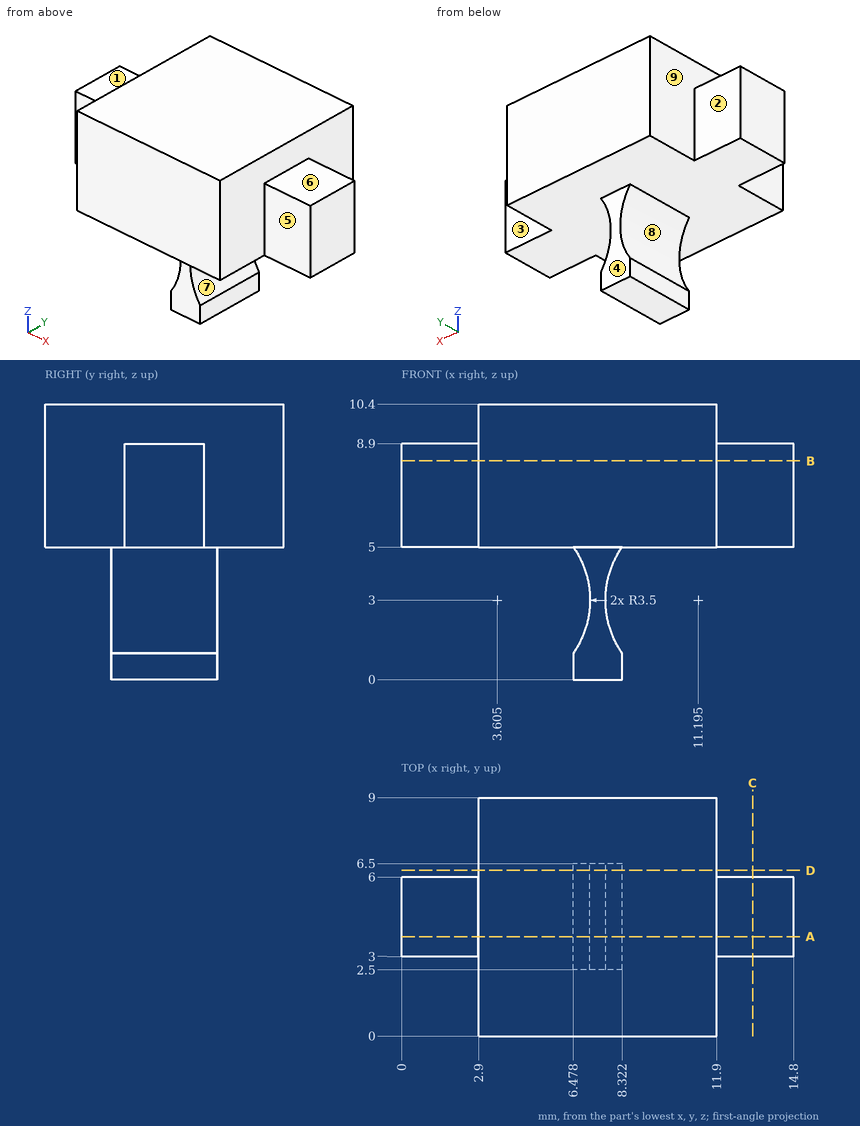
Geometry: see drawing. Coordinates: mm, zero at the bounding-box minimum. A direction names the side the tool comes from. Round coordinates to 2 decimals unless told otherwise and drop trailing zeros. Write each loop counter-clockwise with the first axis right and the second up, starting at its lowest first coordinate (ties: lowest second). Pieces come first, ordered by that corner, then holes.
1) Contact query for flat-ended pins moving along their axis: P1, Ø0.5, axis at y = 3.5, z = 0.5, coming from the -X side; P2, Ø3, axis at x = 1, y = 4.5, coming from the +Z side; P3, Ø0.9, axis at x = 8, z = 3.5, coming from the +Y side. Output: stop coordinate, or through.
2) Reachability of the marked faces 1, 2, 3, 4 and 5 from +Z, -Z, +X, -X, +Y, -Y: full face, straight path, thin tool, end or side. Return the list, or none.
3) Cut plane D-D (y = 6.25). Return the cut outline in (x, z) (1 decimal).
4) Cut plane A-A (y = 3.75). Return the cut outline in (x, z) (1 decimal).
5) Cut plane B-B (z = 8.25). Return the cut outline in (x, y), then the cut area to 3 significant figures.
6) Cut plane C-C (x = 13.25). Return the cut outline in (y, z).
7) Draft query along Z for the marked faces 6, 7, 8 and 9. Return one class per face: pulls with the +Z half, pulls with the -Z half, needs draft (parallel to the pull), parting line crosses it, or undercut.
8) Ray query, L1, parallel to Z at x = 9, y = 4; L2, parallel to X at y = 8, z = 5.5; L3, parallel to X at y = 5.5, z = 3.75 (1 decimal). Return the intervals inside material, ascending.
Geometry says:
1. P1: stops at x = 6.48
1. P2: stops at z = 8.9
1. P3: stops at y = 6.5
2. face 1: +Z, -X, +Y, -Y
2. face 2: +Z, -Z, -X, +Y
2. face 3: +Z, -Z, +X, +Y
2. face 4: -Z, +X, -X, +Y
2. face 5: +Z, -Z, +X, -Y
3. outline: (2.9, 5) - (6.5, 5) arc R3.5 cw to (6.5, 1) - (6.5, 0) - (8.3, 0) - (8.3, 1) arc R3.5 cw to (8.3, 5) - (11.9, 5) - (11.9, 10.4) - (2.9, 10.4) - close
4. outline: (0, 5) - (6.5, 5) arc R3.5 cw to (6.5, 1) - (6.5, 0) - (8.3, 0) - (8.3, 1) arc R3.5 cw to (8.3, 5) - (14.8, 5) - (14.8, 8.9) - (11.9, 8.9) - (11.9, 10.4) - (2.9, 10.4) - (2.9, 8.9) - (0, 8.9) - close
5. outline: (0, 3) - (2.9, 3) - (2.9, 0) - (11.9, 0) - (11.9, 3) - (14.8, 3) - (14.8, 6) - (11.9, 6) - (11.9, 9) - (2.9, 9) - (2.9, 6) - (0, 6) - close
5. area: 98.4 mm2
6. outline: (3, 5) - (6, 5) - (6, 8.9) - (3, 8.9) - close
7. face 6: pulls with the +Z half
7. face 7: undercut
7. face 8: undercut
7. face 9: needs draft
8. L1: z = 5 to 10.4
8. L2: x = 2.9 to 11.9
8. L3: x = 7 to 7.8
